Input: dimensioned drawing with shaded views. Units: mm. Origin: part minimum x, y, z. Round coordinates to 2 decimals unless told otherwise and drop trailing zeros. Order: outer loops, then holes, each group sorted by start corner. A loop starts at its lowest first (then second) coordinate and runs counter-clockwise, first axis right, second up. Notation, with made-up numbers: M -11,65 L 1,65 A18 ccw 1,92 Z; hole C 1,86.25 d2. An arc over 180 degrees is marked long. Answer as CSV lines item,"result". Start each with the question number.
Item 1: Section query D-D on x = 5. Return the cut outline in (y, z).
Item 2: Line query: line 1 (X direction, y = 54, z = 5.5); line 2 (Y direction, x = 5, z = 7.65); line 3 (Y direction, x = 47.5, z = 7). Output: solid intervals per line, ascending. Write a range as [from, to].
Item 3: Pull-direction query (X, two-part tool) for the marked faces 1, 2, 3 and 4; classes: +X half, -X half, draft (parallel to the pull), parting line (faces both ways), or undercut.
Item 4: Section query C-C on x = 49. Return the cut outline in (y, z).
Item 5: First-contact query: P1, Ø3, axis at x = 75, y = 54, coming from the +Z side; P2, Ø12, axis at x = 16.5, y = 6.5, coming from the -Z side; P3, Ø1.5, axis at x = 26.5, z = 4, coming from the -Y side; P4, Ø2.5, axis at x = 54, z = 3.5, coming from the -Y side. Flat tips, straight axial feed; report the tip coordinate or a pass-through.
Item 6: Section query B-B on z = 7. Return the cut outline in (x, y).
Item 7: Section query A-A on y = 54. Return the cut outline in (x, z), plus the area to 3 significant figures.
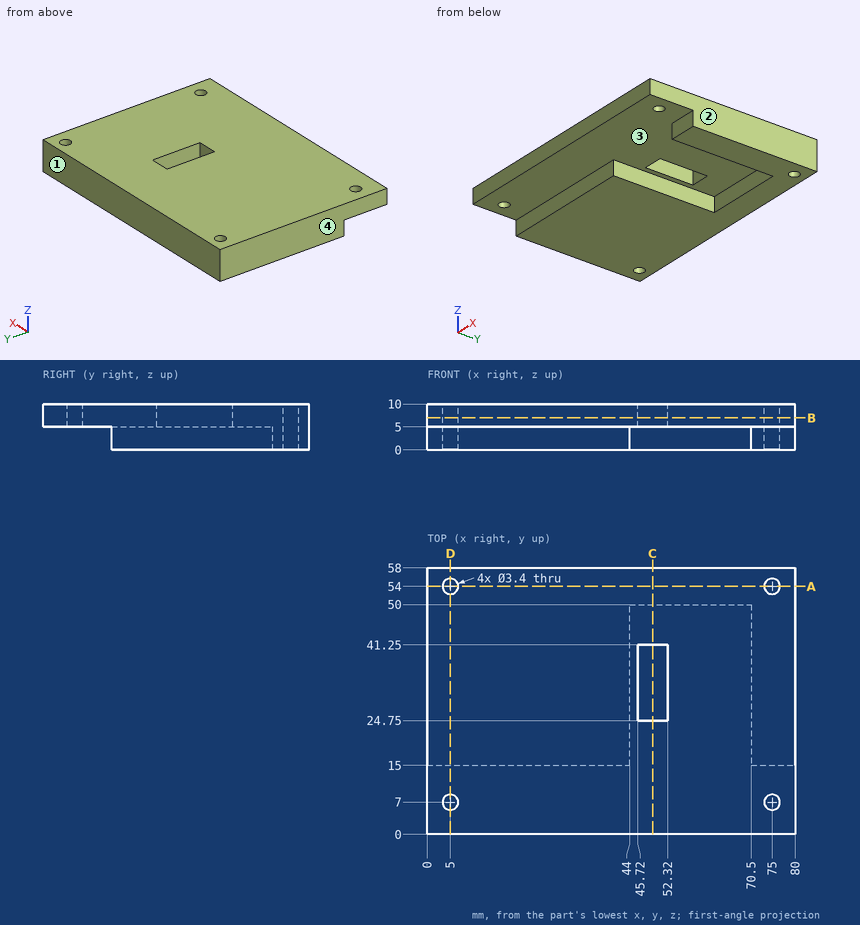
Results:
1,outline,"M 0,5 L 5.3,5 L 5.3,10 L 0,10 Z; M 8.7,5 L 15,5 L 15,0 L 52.3,0 L 52.3,10 L 8.7,10 Z; M 55.7,0 L 58,0 L 58,10 L 55.7,10 Z"
2,line 1,"[0, 3.3], [6.7, 73.3], [76.7, 80]"
2,line 2,"[0, 5.3], [8.7, 52.3], [55.7, 58]"
2,line 3,"[0, 24.75], [41.25, 58]"
3,face 1,"draft"
3,face 2,"+X half"
3,face 3,"undercut"
3,face 4,"-X half"
4,outline,"M 0,5 L 24.75,5 L 24.75,10 L 0,10 Z; M 41.25,5 L 50,5 L 50,0 L 58,0 L 58,10 L 41.25,10 Z"
5,P1,"through"
5,P2,"z = 5"
5,P3,"y = 15"
5,P4,"y = 50"
6,outline,"M 0,0 L 80,0 L 80,58 L 0,58 Z; hole C 5,7 d3.4; hole C 5,54 d3.4; hole M 45.72,24.75 L 52.32,24.75 L 52.32,41.25 L 45.72,41.25 Z; hole C 75,7 d3.4; hole C 75,54 d3.4"
7,outline,"M 0,0 L 3.3,0 L 3.3,10 L 0,10 Z; M 6.7,0 L 73.3,0 L 73.3,10 L 6.7,10 Z; M 76.7,0 L 80,0 L 80,10 L 76.7,10 Z"
7,area,"732 mm^2"
